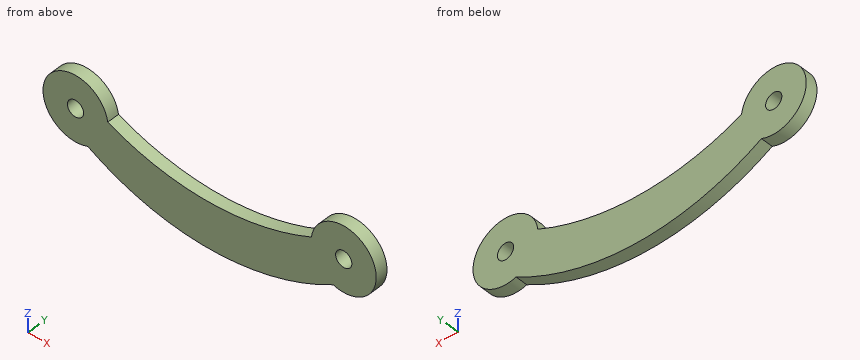
from build123d import *

# Parameters (mm, degrees)
BOSS_EXTRUDE1_DEPTH = 1.5
SKETCH3_R           = 1
CUT_EXTRUDE1_DEPTH  = 11.5


with BuildPart() as part:
    # Sketch1 → Boss-Extrude1 (new body)
    with BuildSketch(Plane(origin=(0, 0, 0), x_dir=(1, 0, 0), z_dir=(0, 1, 0))):
        with BuildLine():
            ThreePointArc((1.506452417, 3.705482575), (-3.464101615, -2), (3.962268252, -0.548115225))
            ThreePointArc((3.962268252, -0.548115225), (16.494990723, 2.195126577), (29.027713195, -0.548115225))
            ThreePointArc((29.027713195, -0.548115225), (36.386316352, -2.207127095), (31.702043975, 3.705482575))
            ThreePointArc((31.702043975, 3.705482575), (16.604248196, 7.78142883), (1.506452417, 3.705482575))
        make_face()
    extrude(amount=BOSS_EXTRUDE1_DEPTH)

    # Sketch3 → Cut-Extrude1 (cut)
    with BuildSketch(Plane(origin=(0, 1.5, 0), x_dir=(1, 0, 0), z_dir=(0, 1, 0))):
        with Locations((33, -0.078075295)):
            Circle(SKETCH3_R)
        Circle(SKETCH3_R)
    extrude(amount=-CUT_EXTRUDE1_DEPTH, mode=Mode.SUBTRACT)


solid = part.part
Work out the finished part from the listing and answer in its coordinate system (mm). Round coordinates to 2 decimals unless told otherwise and drop trailing zeros. Write each loop counter-clockwise with the first axis right and the second up, starting at its lowest first coordinate (ties: lowest second). Pieces come first, ordered by that corner, then holes. Notation, with made-up numbers: M 40,22.25 L 76,22.25 A30 cw 76,55.25 Z; hole C 32.5,-27 d2. An arc over 180 degrees is marked long. Use a Markdown table: item, result.
1) Consider line 1 (X direction, y = 0.9, z = 0); line 2 (Z direction, x = 33, y = 0.65); line 3 (Z direction, x = 0, y = 0.3). Determine where each line is inside the solid, lowest interval first. Write a range as [from, to].
Taken from the geometry:
| item | result |
|---|---|
| line 1 | x = [-4, -1], [1, 5.23], [27.76, 32], [34, 37] |
| line 2 | z = [-3.92, -0.92], [1.08, 4.08] |
| line 3 | z = [-4, -1], [1, 4] |
2) The part is cut by section D-D on x = 10. Give the vertices of the cut face in (y, z).
Taken from the geometry:
| item | result |
|---|---|
| outline | M 0,-7.05 L 1.5,-7.05 L 1.5,-1.48 L 0,-1.48 Z |
3) The part is cut by section B-B on z = 2. Give the vertices of the cut face in (x, y).
Taken from the geometry:
| item | result |
|---|---|
| outline | M -3.46,0 L 3.46,0 L 3.46,1.5 L -3.46,1.5 Z; M 29.49,0 L 36.51,0 L 36.51,1.5 L 29.49,1.5 Z |
4) The part is cut by section C-C on y = 0.95. Give the vertices of the cut face in (x, z) (3 decimals).
Taken from the geometry:
| item | result |
|---|---|
| outline | M 1.506,-3.705 A30 ccw 31.702,-3.705 A4 ccw long 29.028,0.548 A30 cw 3.962,0.548 A4 ccw long Z; hole C 0,0 d2; hole C 33,0.078 d2 |
5) The part is cut by section A-A on x = 33. Give the vertices of the cut face in (y, z), plus the area to 3 significant figures.
Taken from the geometry:
| item | result |
|---|---|
| outline | M 0,-3.92 L 1.5,-3.92 L 1.5,-0.92 L 0,-0.92 Z; M 0,1.08 L 1.5,1.08 L 1.5,4.08 L 0,4.08 Z |
| area | 9.00 mm2 |
